```python
from build123d import *

# Parameters (mm, degrees)
SKETCH2_W               = 120
SKETCH2_H               = 70
BOSS_EXTRUDE1_DEPTH     = 3
SKETCH3_W               = 10
SKETCH3_H               = 3
CUT_EXTRUDE1_DEPTH      = 70.526973183
LPATTERN1_COUNT         = 2
LPATTERN1_PITCH         = 20.5
SKETCH4_W               = 10
SKETCH4_H               = 10
CUT_EXTRUDE2_DEPTH      = 70.526973183
MIRROR1_COPY_1_SKETCH_W = 10
MIRROR1_COPY_1_SKETCH_H = 3
MIRROR1_COPY_1_DEPTH    = 70.526973183
MIRROR2_COPY_1_SKETCH_W = 10
MIRROR2_COPY_1_SKETCH_H = 3
MIRROR2_COPY_1_DEPTH    = 70.526973183
MIRROR2_COPY_2_SKETCH_W = 10
MIRROR2_COPY_2_SKETCH_H = 3
MIRROR2_COPY_2_DEPTH    = 70.526973183
MIRROR2_COPY_3_SKETCH_W = 10
MIRROR2_COPY_3_SKETCH_H = 10
MIRROR2_COPY_3_DEPTH    = 70.526973183
MIRROR2_COPY_4_SKETCH_W = 10
MIRROR2_COPY_4_SKETCH_H = 3
MIRROR2_COPY_4_DEPTH    = 70.526973183


with BuildPart() as part:
    # Sketch2 → Boss-Extrude1 (new body)
    with BuildSketch(Plane.XY):
        Rectangle(SKETCH2_W, SKETCH2_H)
    extrude(amount=BOSS_EXTRUDE1_DEPTH)

    # Sketch3 → Cut-Extrude1 (cut, symmetric)
    with BuildSketch(Plane(origin=(0, 0, 0), x_dir=(-1, 0, 0), z_dir=(0, 0, -1))):
        with Locations((-50, 33.5)):
            Rectangle(SKETCH3_W, SKETCH3_H)
    cut_extrude1 = extrude(amount=CUT_EXTRUDE1_DEPTH, both=True, mode=Mode.SUBTRACT)

    # LPattern1: Cut-Extrude1 ×2
    with Locations(*[(0, -i * LPATTERN1_PITCH, 0) for i in range(1, LPATTERN1_COUNT)]):
        add(cut_extrude1, mode=Mode.SUBTRACT)

    # Sketch4 → Cut-Extrude2 (cut, through all)
    with BuildSketch(Plane(origin=(0, 0, 0), x_dir=(-1, 0, 0), z_dir=(0, 0, -1))):
        with Locations((-33, 27)):
            Rectangle(SKETCH4_W, SKETCH4_H)
    cut_extrude2 = extrude(amount=-CUT_EXTRUDE2_DEPTH, mode=Mode.SUBTRACT)

    # Mirror1: Cut-Extrude1, Cut-Extrude2 across plane
    add(cut_extrude1.mirror(Plane.ZX), mode=Mode.SUBTRACT)
    add(cut_extrude2.mirror(Plane.ZX), mode=Mode.SUBTRACT)

    # Mirror1 copy 1 sketch → Mirror1 copy 1 (cut, symmetric)
    with BuildSketch(Plane(origin=(0, 20.5, 0), x_dir=(-1, 0, 0), z_dir=(0, 0, -1))):
        with Locations((-50, -33.5)):
            Rectangle(MIRROR1_COPY_1_SKETCH_W, MIRROR1_COPY_1_SKETCH_H)
    extrude(amount=MIRROR1_COPY_1_DEPTH, both=True, mode=Mode.SUBTRACT)

    # Mirror2: Cut-Extrude1, Cut-Extrude2 across plane
    add(cut_extrude1.mirror(Plane(origin=(0, 0, 0), x_dir=(0, 0, 1), z_dir=(1, 0, 0))), mode=Mode.SUBTRACT)
    add(cut_extrude2.mirror(Plane(origin=(0, 0, 0), x_dir=(0, 0, 1), z_dir=(1, 0, 0))), mode=Mode.SUBTRACT)

    # Mirror2 copy 1 sketch → Mirror2 copy 1 (cut, symmetric)
    with BuildSketch(Plane(origin=(0, -20.5, 0), x_dir=(1, 0, 0), z_dir=(0, 0, -1))):
        with Locations((-50, -33.5)):
            Rectangle(MIRROR2_COPY_1_SKETCH_W, MIRROR2_COPY_1_SKETCH_H)
    extrude(amount=MIRROR2_COPY_1_DEPTH, both=True, mode=Mode.SUBTRACT)

    # Mirror2 copy 2 sketch → Mirror2 copy 2 (cut, symmetric)
    with BuildSketch(Plane(origin=(0, 0, 0), x_dir=(1, 0, 0), z_dir=(0, 0, -1))):
        with Locations((-50, 33.5)):
            Rectangle(MIRROR2_COPY_2_SKETCH_W, MIRROR2_COPY_2_SKETCH_H)
    extrude(amount=MIRROR2_COPY_2_DEPTH, both=True, mode=Mode.SUBTRACT)

    # Mirror2 copy 3 sketch → Mirror2 copy 3 (cut, through all)
    with BuildSketch(Plane(origin=(0, 0, 0), x_dir=(1, 0, 0), z_dir=(0, 0, -1))):
        with Locations((-33, 27)):
            Rectangle(MIRROR2_COPY_3_SKETCH_W, MIRROR2_COPY_3_SKETCH_H)
    extrude(amount=-MIRROR2_COPY_3_DEPTH, mode=Mode.SUBTRACT)

    # Mirror2 copy 4 sketch → Mirror2 copy 4 (cut, symmetric)
    with BuildSketch(Plane(origin=(0, 20.5, 0), x_dir=(1, 0, 0), z_dir=(0, 0, -1))):
        with Locations((-50, 33.5)):
            Rectangle(MIRROR2_COPY_4_SKETCH_W, MIRROR2_COPY_4_SKETCH_H)
    extrude(amount=MIRROR2_COPY_4_DEPTH, both=True, mode=Mode.SUBTRACT)


solid = part.part
```
The listing builds one solid part. Answer for the finished solid, in the listing's coordinates (mm). A direction names the side the tool comes from. Give positions to 0.01 mm unless a question says otherwise; leave off trailing zeros. Loops run counter-clockwise (first coordinate to the right, second up) from the corner with the lowest first, then second, coordinate; pieces in that order, holes last. Notation, with made-up numbers: (64, -10.75) - (79, -10.75) arc R8 cw to (79, -0.75) - close; hole circle Ø9 at (45.25, -3). An arc over 180 degrees is marked (long way). Answer as CSV lines item,"result". Start each with the question number.
Item 1: For faces 1 (the face through (57, 35, 1)), 2 (the face through (50, 32, 1)), 3 (the face through (-50, 14.5, 1)), 4 (the face through (-1, 0, 0)), 5 (the face through (-50, -32, 1)), determine the directions among +Z, -Z, +X, -X, +Y, -Y from which every point of the face is accessible in a straight line to the end or side of a thin tool.
Item 2: A cutting plane is placed at C-C on z = 0.6. Count the separate pieces of the cut face and the enclosed holes in it, then the cut area to 3 significant figures.
Item 3: Find the intervals of material crossed by line 1 (X direction, y = 28, z = 0.4); line 2 (Y direction, x = 54.5, z = 1.4); line 3 (Y direction, x = 34, z = 0.9), in increasing order. Write a range as from..to.
Item 4: The mould has two halves that part along X. Classify faces 6 (the face through (-60, 0, 1)), 7 (the face through (57, -35, 1)), 8 (the face through (-33, -22, 1)): +X half, -X half, draft (parallel to the pull), parting line (faces both ways), or undercut.
Item 5: A cutting plane is placed at A-A on x = 33. Determine the outline of the cut face in (y, z), then the cut area to 3 significant figures.
Item 6: This flat-tipped pin is pushed along its axis until it touches: pin 1 (8 mm diameter, centred on x = -36, y = -3.5, fed in from -Z). Where does it stop, or does it pass through?
Item 7: A cutting plane is placed at B-B on x = -47. Determine the outline of the cut face in (y, z).
Found:
1,face 1,"+Z, -Z, +X, -X, +Y"
1,face 2,"+Z, -Z, +Y"
1,face 3,"+Z, -Z"
1,face 4,"-Z, +X, -X, +Y, -Y"
1,face 5,"+Z, -Z, -Y"
2,separate pieces,"1"
2,enclosed holes,"8"
2,area,"7,760 mm^2"
3,line 1,"x = -60..-38, -28..28, 38..60"
3,line 2,"y = -32..-14.5, -11.5..11.5, 14.5..32"
3,line 3,"y = -35..-32, -22..22, 32..35"
4,face 6,"-X half"
4,face 7,"draft"
4,face 8,"undercut"
5,outline,"(-35, 0) - (-32, 0) - (-32, 3) - (-35, 3) - close; (-22, 0) - (22, 0) - (22, 3) - (-22, 3) - close; (32, 0) - (35, 0) - (35, 3) - (32, 3) - close"
5,area,"150 mm^2"
6,pin 1,"stops at z = 0"
7,outline,"(-32, 0) - (-14.5, 0) - (-14.5, 3) - (-32, 3) - close; (-11.5, 0) - (11.5, 0) - (11.5, 3) - (-11.5, 3) - close; (14.5, 0) - (32, 0) - (32, 3) - (14.5, 3) - close"
